Geometry check sheet. Reference: drawing and pictorial views, mm from the part's lowest x, y, z. Coordinates: 2 decimals unless noted, no trailing zeros. Loops run counter-clockwise (first coordinate to the right, second up) from the corner with the lowest first, then second, coordinate; pieces in that order, holes last. Notation, with made-up numbers: (16, 80.25) -> (31, 80.25) arc R5 ccw to (31, 89.25) -> close; hole circle Ø6 at (76.25, 14). An arc over 180 degrees is marked (long way). Use one line per item in the form item = value.
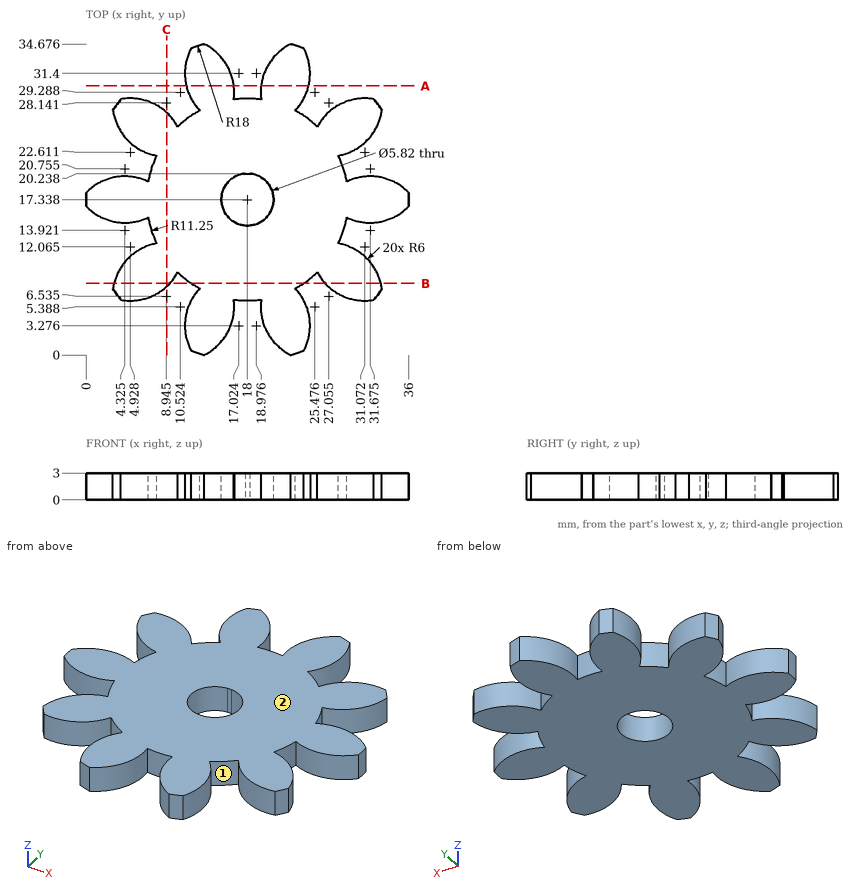
(1) Section check C-C, the plane x = 9. Record the boundary of the cut face in (y, z).
Established:
outline = (7.66, 0) -> (27.02, 0) -> (27.02, 3) -> (7.66, 3) -> close
(2) Scan lines: line 1 along Y through (x, z) = (18, 1.2); line 2 along X through (y, z) = (8, 1.65) (1 decimal); line 3 along X through (y, z) = (28, 2.6) (1 decimal). Record each from-to range of solid material in increasing order.
Established:
line_1 = 6.09 to 14.43, 20.24 to 28.59
line_2 = 3.1 to 9.3, 11.7 to 24.3, 26.7 to 32.9
line_3 = 3.5 to 7.6, 12.1 to 23.9, 28.4 to 32.5
(3) Mould release check, pull along X, two halves, no side actions. Record for the marked faces 1 and 2: +X half, -X half, draft (parallel to the pull), parting line (faces both ways), or undercut.
Established:
face_1 = undercut
face_2 = draft
(4) Go/stop test with flat-tipped pins: P1, Ø1.5, axis at x = 28.5, z = 1.5, coming from the +Y side; P2, Ø8, axis at x = 6, y = 22, coming from the +Z side; P3, Ø1.5, axis at x = 26, z = 0.5, coming from the -Y side. Record where each tip stops, or that it passes through.
Established:
P1 = 28.33
P2 = 3
P3 = 7.9
(5) Section check B-B, the plane y = 8. Record the boundary of the cut face in (x, z) (1 decimal).
Established:
outline = (3.1, 0) -> (9.3, 0) -> (9.3, 3) -> (3.1, 3) -> close; (11.7, 0) -> (24.3, 0) -> (24.3, 3) -> (11.7, 3) -> close; (26.7, 0) -> (32.9, 0) -> (32.9, 3) -> (26.7, 3) -> close
(6) Section check A-A, the plane y = 30. Record the boundary of the cut face in (x, z).
Established:
outline = (11.19, 0) -> (16.48, 0) -> (16.48, 3) -> (11.19, 3) -> close; (19.52, 0) -> (24.81, 0) -> (24.81, 3) -> (19.52, 3) -> close
